Geometry check sheet. Reference: the model listing, model coordinates, mm. Face numbers are marked on the shaded views. A direction names the side the tool comes from. Round coordinates to 2 decimals unless told otherwise and drop trailing zeros. Write each loop counter-clockwise with the first axis right and the second up, starting at its lowest first coordinate (ties: lowest second). Pieces come first, ordered by that corner, then holes. Notation, with made-up numbers: (-11, 46) -> (46, 46) arc R31 ccw to (46, 81) -> close; hole circle Ø7 at (63.25, 80). An arc over 180 degrees is marked (long way). Return JSON: item names as keys, results as strings. Group by question number.
from build123d import *

# Parameters (mm, degrees)
F0_R     = 6.35
F1_DEPTH = 38.1
F3_D     = 5
F3_DEPTH = 15.001
F5_D     = 3
F5_DEPTH = 29.501
F6_R     = 10


with BuildPart() as f1:
    # F0 (on Top) → F1 (new body)
    with BuildSketch(Plane.XY):
        with BuildLine():
            ThreePointArc((-18.4282391997, -40.45), (-43.9709210804, -6.508502081), (-29.3559965753, 33.3770574658))
            Line((-29.3559965753, 33.3770574658), (-29.3559965753, 45.4292414335))
            Line((-29.3559965753, 45.4292414335), (29.3559965753, 45.4292414335))
            Line((29.3559965753, 45.4292414335), (29.3559965753, 33.3770574658))
            ThreePointArc((29.3559965753, 33.3770574658), (38.0001883545, -23.0605330603), (-16.0530370958, -41.45))
            Line((-16.0530370958, -41.45), (-56.45, -41.45))
            Line((-56.45, -41.45), (-56.45, -56.45))
            Line((-56.45, -56.45), (56.45, -56.45))
            Line((56.45, -56.45), (56.45, 57.4292414335))
            Line((56.45, 57.4292414335), (28, 57.4292414335))
            Line((28, 57.4292414335), (28, 60.4292414335))
            Line((28, 60.4292414335), (-32, 60.4292414335))
            Line((-32, 60.4292414335), (-32, 57.4292414335))
            Line((-32, 57.4292414335), (-56.45, 57.4292414335))
            Line((-56.45, 57.4292414335), (-56.45, -26.95))
            Line((-56.45, -26.95), (-49.6300168369, -26.95))
            Line((-49.6300168369, -26.95), (-49.6300168369, -32.45))
            Line((-49.6300168369, -32.45), (-56.45, -32.45))
            Line((-56.45, -32.45), (-56.45, -40.45))
            Line((-56.45, -40.45), (-18.4282391997, -40.45))
        make_face()
        with Locations((44.45, -44.45)):
            Circle(F0_R, mode=Mode.SUBTRACT)
    extrude(amount=F1_DEPTH)

    # F3 (through all, one way)
    with BuildSketch(Plane.XZ.offset(-45.4292414335)):
        with Locations((-19.3559965753, 25.4), (-19.3559965753, 12.7), (20.6440034247, 25.4), (20.6440034247, 12.7), (0, 25.4), (0, 12.7)):
            Circle(F3_D / 2)
    extrude(amount=-F3_DEPTH, mode=Mode.SUBTRACT)

    # F5 (through all, one way)
    with BuildSketch(Plane(origin=(0, -26.95, 0), x_dir=(1, 0, 0), z_dir=(0, 1, 0))):
        with Locations((-53.0400084184, -25.4), (-53.0400084184, -12.7)):
            Circle(F5_D / 2)
    extrude(amount=-F5_DEPTH, mode=Mode.SUBTRACT)

    # F6
    f6_edges = [f1.edges().sort_by_distance(p)[0] for p in [
        (56.45, 57.429241, 19.05),
        (-56.45, 57.429241, 19.05),
        (56.45, -56.45, 19.05),
    ]]
    fillet(f6_edges, radius=F6_R)


solid = f1.part
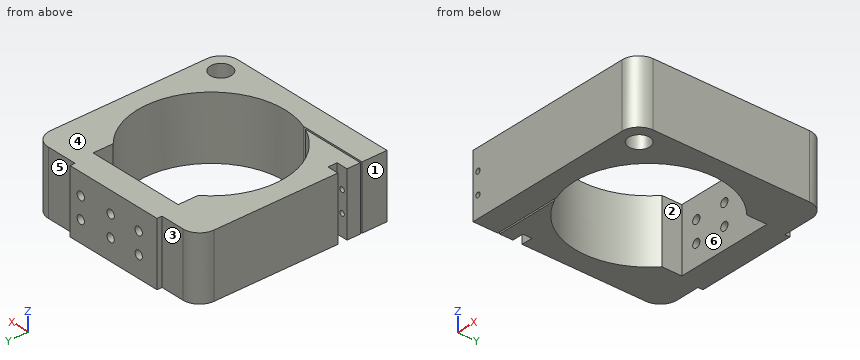
1) Sectioned sample at B-B on z = 20.5. Enter the section's corners in (x, y).
2) Tool access check on the marked faces 4, 5 and 6. Record the directions out of +Z, -Z, +X, -X, +Y, -Y that give a thin tool (end or side, any length) a straight path to the whole face; none if there is none.
3) Material ranges on probe 1 along Z at (x, y) = (0, 49.5); probe 2 along X at (y, z) = (-1, 33.5); probe 3 along Y at (x, z) = (-20.5, 36.5), recorded low to high. Write a range as [from, to].
4) Sectioned sample at A-A on y = -34. Enter the section's corners in (x, z).
5) Sectioned sample at D-D on y = 35. Enter the section's corners in (x, z), and give its area (3 significant figures).
6) Sectioned sample at C-C on x = 0. Enter the section's corners in (y, z).
7) Go/stop test with flat-tipped pins: P1, Ø5.5, axis at x = -52, z = 15.5, coming from the +Y side; P2, Ø4, axis at x = 20.64, z = 12.7, coming from the +Y side; P3, Ø1.5, axis at y = 59.5, z = 27.5, coming from the -X side. Record where each tip stops, or that it passes through.
8) Mould release check, pull along Y, two halves, no side actions. Record for the marked faces 1, 2 and 3: +Y half, -Y half, draft (parallel to the pull), parting line (faces both ways), or undercut.
Evaluation:
{
 "1": {"outline": "(-56.45, -56.45) -> (46.45, -56.45) arc R10 ccw to (56.45, -46.45) -> (56.45, 47.43) arc R10 ccw to (46.45, 57.43) -> (28, 57.43) -> (28, 60.43) -> (-32, 60.43) -> (-32, 57.43) -> (-46.45, 57.43) arc R10 ccw to (-56.45, 47.43) -> (-56.45, -26.95) -> (-49.63, -26.95) -> (-49.63, -32.45) -> (-56.45, -32.45) -> (-56.45, -40.45) -> (-18.43, -40.45) arc R44.45 cw to (-29.36, 33.38) -> (-29.36, 45.43) -> (29.36, 45.43) -> (29.36, 33.38) arc R44.45 cw to (-16.05, -41.45) -> (-56.45, -41.45) -> close; hole circle Ø12.7 at (44.45, -44.45)"},
 "2": {"face 4": "+Z, +X, -X, +Y, -Y", "face 5": "+Z, -Z, +X, +Y", "face 6": "+Z, -Z"},
 "3": {"probe 1": "z = [0, 10.2], [15.2, 22.9], [27.9, 38.1]", "probe 2": "x = [-56.45, -44.44], [44.44, 56.45]", "probe 3": "y = [-56.45, -41.45], [-40.45, -39.44], [45.43, 60.43]"},
 "4": {"outline": "(-56.45, 0) -> (-28.63, 0) -> (-28.63, 38.1) -> (-56.45, 38.1) -> close; (28.63, 0) -> (56.45, 0) -> (56.45, 38.1) -> (28.63, 38.1) -> close; hole circle Ø3 at (-53.04, 12.7); hole circle Ø3 at (-53.04, 25.4)"},
 "5": {"outline": "(-56.45, 0) -> (-29.36, 0) -> (-29.36, 38.1) -> (-56.45, 38.1) -> close; (29.36, 0) -> (56.45, 0) -> (56.45, 38.1) -> (29.36, 38.1) -> close", "area": "2,060 mm2"},
 "6": {"outline": "(-56.45, 0) -> (-44.45, 0) -> (-44.45, 38.1) -> (-56.45, 38.1) -> close; (45.43, 0) -> (60.43, 0) -> (60.43, 10.2) -> (45.43, 10.2) -> close; (45.43, 15.2) -> (60.43, 15.2) -> (60.43, 22.9) -> (45.43, 22.9) -> close; (45.43, 27.9) -> (60.43, 27.9) -> (60.43, 38.1) -> (45.43, 38.1) -> close"},
 "7": {"P1": "stops at y = 57.03", "P2": "stops at y = -38.25", "P3": "stops at x = -32"},
 "8": {"face 1": "draft", "face 2": "undercut", "face 3": "+Y half"}
}
